Autodesk Inventor part; units mm, degrees
ref_plane "YZ Plane" through (0, 0, 0) normal (1, 0, 0) x (0, 1, 0)
ref_plane "XZ Plane" through (0, 0, 0) normal (0, 1, 0) x (-1, 0, 0)
ref_plane "XY Plane" through (0, 0, 0) normal (0, 0, 1) x (1, 0, 0)
sketch "Sketch1" plane through (0, 0, 0) normal (0, 1, 0) x (-1, 0, 0)
  circle A0 centre (0, 0) radius 114.3
  dimension "d0" = 228.6
extrude "Extrusion1" add sketch "Sketch1" along normal blind 7.9756
sketch "Sketch2" plane through (0, 7.9756, 0) normal (0, 1, 0) x (1, 0, 0)
  circle A0 centre (0, 0) radius 114.3
  circle A1 centre (0, 0) radius 74.2569
  dimension "d3" = 148.5138
extrude "Extrusion2" add sketch "Sketch2" along normal blind 41.0464 contours A1
sketch "Sketch3" plane through (0, 49.022, 0) normal (0, 1, 0) x (1, 0, 0)
  circle A0 centre (0, 0) radius 74.2569
  circle A1 centre (0, 0) radius 114.3
  dimension "d6" = 228.6
extrude "Extrusion3" add sketch "Sketch3" along normal blind 7.9756 contours A0 | A1
sketch "Sketch4" plane through (0, 56.9976, 0) normal (0, 1, 0) x (1, 0, 0)
  circle A0 centre (0, 0) radius 114.3
  circle A1 centre (0, 0) radius 111.76
  circle A2 centre (0, 0) radius 74.2569
  line L0 (14.605, 72.8065) -> (7.62, 111.4999)
  line L1 (-14.605, 72.8065) -> (-7.62, 111.4999)
  line L2 (0, 0) -> (0, 82.3144)
  circle A3 centre (0, 0) radius 111.76
  circle A4 centre (0, 0) radius 74.2569
  line L3 (-23.7549, 70.3547) -> (-49.1508, 100.3718)
  line L4 (-49.0515, 55.7497) -> (-62.3491, 92.7518)
  circle A5 centre (0, 0) radius 111.76
  circle A6 centre (0, 0) radius 74.2569
  line L5 (-55.7497, 49.0515) -> (-92.7518, 62.3491)
  line L6 (-70.3547, 23.7549) -> (-100.3718, 49.1508)
  circle A7 centre (0, 0) radius 111.76
  circle A8 centre (0, 0) radius 74.2569
  line L7 (-72.8065, 14.605) -> (-111.4999, 7.62)
  line L8 (-72.8065, -14.605) -> (-111.4999, -7.62)
  circle A9 centre (0, 0) radius 111.76
  circle A10 centre (0, 0) radius 74.2569
  line L9 (-70.3547, -23.7549) -> (-100.3718, -49.1508)
  line L10 (-55.7497, -49.0515) -> (-92.7518, -62.3491)
  circle A11 centre (0, 0) radius 111.76
  circle A12 centre (0, 0) radius 74.2569
  line L11 (-49.0515, -55.7497) -> (-62.3491, -92.7518)
  line L12 (-23.7549, -70.3547) -> (-49.1508, -100.3718)
  circle A13 centre (0, 0) radius 111.76
  circle A14 centre (0, 0) radius 74.2569
  line L13 (-14.605, -72.8065) -> (-7.62, -111.4999)
  line L14 (14.605, -72.8065) -> (7.62, -111.4999)
  circle A15 centre (0, 0) radius 111.76
  circle A16 centre (0, 0) radius 74.2569
  line L15 (23.7549, -70.3547) -> (49.1508, -100.3718)
  line L16 (49.0515, -55.7497) -> (62.3491, -92.7518)
  circle A17 centre (0, 0) radius 111.76
  circle A18 centre (0, 0) radius 74.2569
  line L17 (55.7497, -49.0515) -> (92.7518, -62.3491)
  line L18 (70.3547, -23.7549) -> (100.3718, -49.1508)
  circle A19 centre (0, 0) radius 111.76
  circle A20 centre (0, 0) radius 74.2569
  line L19 (72.8065, -14.605) -> (111.4999, -7.62)
  line L20 (72.8065, 14.605) -> (111.4999, 7.62)
  circle A21 centre (0, 0) radius 111.76
  circle A22 centre (0, 0) radius 74.2569
  line L21 (70.3547, 23.7549) -> (100.3718, 49.1508)
  line L22 (55.7497, 49.0515) -> (92.7518, 62.3491)
  circle A23 centre (0, 0) radius 111.76
  circle A24 centre (0, 0) radius 74.2569
  line L23 (49.0515, 55.7497) -> (62.3491, 92.7518)
  line L24 (23.7549, 70.3547) -> (49.1508, 100.3718)
  dimension "d10" = 148.5138
  dimension "d11" = 29.21
  dimension "d12" = 14.605
  dimension "d13" = 15.24
  dimension "d14" = 7.62
  dimension "d17" = 360
extrude "Extrusion4" cut sketch "Sketch4" against normal blind 12700 contours A1 L19 A2 L20 | L21 A2 L22 A1 | A1 L17 A2 L18 | L23 A2 L24 A1 | A1 L13 A2 L14 | A1 L11 A2 L12 | A1 L9 A2 L10 | L7 A2 L8 A1
sketch "Sketch5" plane through (0, 56.9976, 0) normal (0, 1, 0) x (1, 0, 0)
  arc A0 (100.3718, 49.1508) -> (92.7518, 62.3491) centre (0, 0) ccw
  circle A1 centre (0, 29.1163) radius 12.7
  circle A2 centre (-27.6912, 8.9974) radius 12.7
  circle A3 centre (-17.1141, -23.5556) radius 12.7
  circle A4 centre (17.1141, -23.5556) radius 12.7
  circle A5 centre (27.6912, 8.9974) radius 12.7
  dimension "d21" = 25.4
  dimension "d24" = 360
extrude "Extrusion5" cut sketch "Sketch5" against normal blind 12700
sketch "Sketch6" plane through (0, 49.022, 0) normal (0, -1, 0) x (1, 0, 0)
  arc A0 (70.3547, -23.7549) -> (72.8065, -14.605) centre (0, 0) ccw
  circle A1 centre (0, 0) radius 70.5777
extrude "Extrusion6" cut sketch "Sketch6" along normal blind 41.021
sketch "Sketch7" plane through (0, 0, 0) normal (0, -1, 0) x (1, 0, 0)
  circle A0 centre (0, 0) radius 114.3
  circle A1 centre (0, 0) radius 7.62
  dimension "d30" = 15.24
extrude "Extrusion7" cut sketch "Sketch7" against normal blind 174.879 contours A1
properties part number "Wheel"
CAD build for the part. Positions are in the model's coordinates, mm. Round coordinates to 2 decimals unless told otherwise and drop trailing zeros. Order: outer loops, then holes, each group sorted by start corner. A loop starts at its lowest first (then second) coordinate and runs counter-clockwise, first axis right, second up. Notation, with made-up numbers: (31, 67.5) - (49, 67.5) arc R31 cw to (49, 98.5) - close; hole circle Ø4 at (46, -11). An arc over 180 degrees is marked (long way). Answer as CSV lines item,"result". Start each with the question number.
1. Saw through at C-C, the plane z = -59. Write the cut outline in (x, y), and give its area (3 significant figures).
2. Saw through at B-B, the plane x = 65. Write the cut outline in (y, z), and give its area (3 significant figures).
3. Pin check, flat tips, straight feed: pin 1 (8 mm diameter, centred on y = 21, z = 72, fed in from +X); pin 2 (6 mm diameter, centred on y = 6.5, z = -47, fed in from -X); pin 3 (5 mm diameter, centred on y = 9.5, z = 64.5, fed in from -X). Stop position of each tip, or through.
4. Drill centre lines: L1, parallel to Y at x = 8.5, z = -62; L2, parallel to X at y = 6, z = 75.5; L3, parallel to X at y = 51, z = -34.5. Where is each one in solid material? Low to high. Write a range as [from, to].
5. Saw through at A-A, the plane z = 18. Count the separate pieces of the cut face and the enclosed holes in it, and give its area (3 significant figures).
6. Pull direction X, two halves, no side cores. Call faces 1 (the face through (1, 7.976, -76)), 2 (the face through (111.76, 53.07, 0.11)): +X half, -X half, draft (parallel to the pull), parting line (faces both ways), or undercut.
Model answer:
1,outline,"(-97.9, 0) - (45.09, 0) - (45.09, 57) - (-97.9, 57) - (-97.9, 49.02) - (-45.09, 49.02) - (-45.09, 7.98) - (-97.9, 7.98) - close; (50.22, 0) - (83.43, 0) - (83.43, 7.98) - (50.22, 7.98) - close; (50.22, 49.02) - (83.43, 49.02) - (83.43, 57) - (50.22, 57) - close; (94.92, 0) - (97.9, 0) - (97.9, 7.98) - (94.92, 7.98) - close; (94.92, 49.02) - (97.9, 49.02) - (97.9, 57) - (94.92, 57) - close; hole (-38.73, 8) - (38.73, 8) - (38.73, 49.02) - (-38.73, 49.02) - close"
1,area,"3,380 mm²"
2,outline,"(0, -94.02) - (7.98, -94.02) - (7.98, -52.38) - (0, -52.38) - close; (0, -35.9) - (57, -35.9) - (57, 35.9) - (0, 35.9) - close; (0, 52.38) - (7.98, 52.38) - (7.98, 94.02) - (0, 94.02) - close; (49.02, -94.02) - (57, -94.02) - (57, -52.38) - (49.02, -52.38) - close; (49.02, 52.38) - (57, 52.38) - (57, 94.02) - (49.02, 94.02) - close; hole (8, -27.5) - (49.02, -27.5) - (49.02, 27.5) - (8, 27.5) - close"
2,area,"3,170 mm²"
3,pin 1,"stops at x = 29.83"
3,pin 2,"stops at x = -105.49"
3,pin 3,"stops at x = -95.69"
4,L1,"y = [0, 8], [49.02, 57]"
4,L2,"x = [-85.82, -56.15], [-28.11, -14.12], [14.12, 85.82]"
4,L3,"x = [-108.97, -11.5], [11.5, 65.76], [83.06, 108.97]"
5,separate pieces,"4"
5,enclosed holes,"0"
5,area,"3,190 mm²"
6,face 1,"draft"
6,face 2,"undercut"
